Model file for the job. Use its own axes, mm. Round coordinates to 2 decimals unless told otherwise and drop trailing zeros. Loops run counter-clockwise (first coordinate to the right, second up) from the corner with the lowest first, then second, coordinate; pieces in that order, holes last.
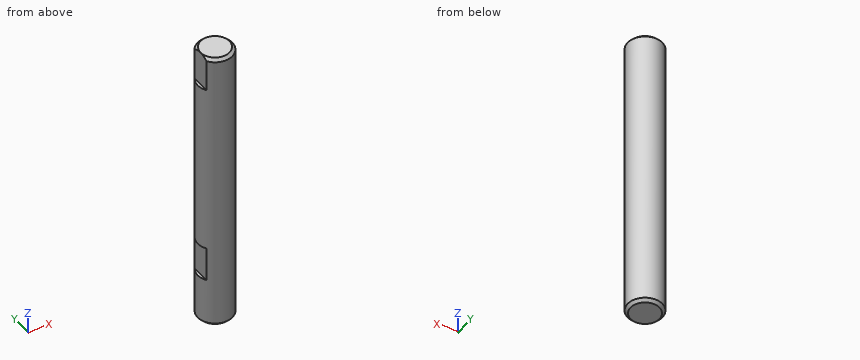
Autodesk Inventor part; units mm, degrees
ref_plane "YZ Plane" through (0, 0, 0) normal (1, 0, 0) x (0, 1, 0)
ref_plane "XZ Plane" through (0, 0, 0) normal (0, 1, 0) x (-1, 0, 0)
ref_plane "XY Plane" through (0, 0, 0) normal (0, 0, 1) x (1, 0, 0)
sketch "Skizze1" plane through (0, 0, 0) normal (0, 0, 1) x (1, 0, 0)
  circle A0 centre (0, 0) radius 3
  dimension "d0" = 6
extrude "Extrusion1" add sketch "Skizze1" along normal blind 8.5
sketch "Skizze2" plane through (0, 0, 8.5) normal (0, 0, 1) x (1, 0, 0)
  circle A0 centre (0, 0) radius 3
  line L0 (-2.5, 1.6583) -> (-2.5, -1.6583)
  dimension "d3" = 2.5
extrude "Extrusion2" add sketch "Skizze2" along normal blind 6 contours A0 L0 picked at (-0.6667, 0)
sketch "Skizze3" plane through (0, 0, 14.5) normal (0, 0, 1) x (1, 0, 0)
  circle A0 centre (0, 0) radius 3
extrude "Extrusion3" add sketch "Skizze3" along normal blind 30
sketch "Skizze4" plane through (0, 0, 44.5) normal (0, 0, 1) x (1, 0, 0)
  line L0 (-2.5, -1.6583) -> (-2.5, 1.6583)
  arc A0 (-2.5, 1.6583) -> (-2.5, -1.6583) centre (0, 0) ccw
  circle A1 centre (0, 0) radius 3
extrude "Extrusion4" add sketch "Skizze4" along normal blind 6 contours L0 A1
chamfer "Fase1" distance 0.5 angle 45 3 edges at (-3, 0, 0) (0.866, -2.8723, 50.5) (0.866, 2.8723, 50.5)
properties part number "Welle_wrist" material "Edelstahl"
Q1. Slice it at A-A on z = 17. Give the cut face in (x, y), plus the area to 3 significant figures.
Q2. Flat gauge pins, fed straight in: P1, Ø0.6, axis at x = -3, y = 0, coming from the +Z side; P2, Ø1.7, axis at y = 0, z = 11.5, coming from the -X side. Where does each tip first touch, or does it go through?
Q3. Probe line 1 (Y direction, x = -0.25, z = 10.5); line 2 (X direction, y = -0.15, z = 9.5); line 3 (Z direction, x = -0.65, y = -2.55). List the from-to ranges inside material, lowest first.
Reply:
1. outline: circle Ø6 at (0, 0)
1. area: 28.3 mm2
2. P1: stops at z = 44.5
2. P2: stops at x = -2.5
3. line 1: y = -2.99 to 2.99
3. line 2: x = -2.5 to 3
3. line 3: z = 0.13 to 50.37
